Part model, mm, in its own coordinate system. Coordinates: 2 decimals unless noted, no trailing zeros. Loops run counter-clockwise (first coordinate to the right, second up) from the corner with the lowest first, then second, coordinate; pieces in that order, holes last. Notation, with made-up numbers: M -37.5,56.25 L 12.5,56.25 A18 cw 12.5,76.25 Z; hole C 32,75 d6. An arc over 180 degrees is marked long. Use a Markdown table: item, result. Add a question column.
1) Band-saw the part on A-A (y = 10). List the corners of the cut face in (x, z), plus the area to 3 significant figures.
2) Pin check, flat tips, straight feed: pin 1 Ø1.5 at (y, z) = (18.5, 2) entering from -X; pin 2 Ø1.5 at (y, z) = (9, 1.5) entering from +X; pin 3 Ø1.8 at (x, y) = (9.91, 15.79) entering from -Z. Stop position of each tip, or through.
3) Wall check: probe 1 along X at (y, z) = (25.25, 1.7); probe 2 along Y at (x, z) = (67.5, 0.1); probe 3 along Y at (x, z) = (19.5, 0.2). Give the ranges that are in metal, low to high. Write a range as from..to.
4) Band-saw the part on B-B (x = 15). List the corners of the cut face in (y, z), plus the area to 3 significant figures.
5) Band-saw the part on C-C (x = 33). List the corners of the cut face in (y, z), plus the area to 3 significant figures.
from build123d import *

# Parameters (mm, degrees)
MODEL_R                 = 1
SALIENTE_EXTRUIR1_DEPTH = 3


with BuildPart() as part:
    # Model → Saliente-Extruir1 (new body)
    with BuildSketch(Plane.XY):
        with BuildLine():
            Line((17.861622063, 18.20706488), (56.277425925, 14.846117598))
            Line((56.277425925, 14.846117598), (67.057874252, 21.223257456))
            ThreePointArc((67.057874252, 21.223257456), (71.209474737, 20.095027087), (69.964368376, 15.976969231))
            Line((69.964368376, 15.976969231), (55.736188762, 8.659748523))
            Line((55.736188762, 8.659748523), (18.934882774, 11.8794456))
            ThreePointArc((18.934882774, 11.8794456), (8.451096418, 6.06231898), (0.138961898, 14.702756365))
            Line((0.138961898, 14.702756365), (-1.772059081, 14.490982222))
            ThreePointArc((-1.772059081, 14.490982222), (-1.880981546, 14.481466547), (-1.990228383, 14.477019049))
            ThreePointArc((-1.990228383, 14.477019049), (-2.005285406, 14.476804272), (-2.020343495, 14.476685822))
            ThreePointArc((-2.020343495, 14.476685822), (-4.376324998, 17.035772608), (-1.611755391, 19.146869222))
            ThreePointArc((-1.611755391, 19.146869222), (-1.596946637, 19.144137761), (-1.582155659, 19.141311623))
            ThreePointArc((-1.582155659, 19.141311623), (-1.475340827, 19.117961178), (-1.369725519, 19.08967588))
            Line((-1.369725519, 19.08967588), (0.550429384, 18.527326068))
            ThreePointArc((0.550429384, 18.527326068), (1.632460158, 18.600931479), (2.408362946, 19.35868026))
            ThreePointArc((2.408362946, 19.35868026), (2.540100184, 19.623117729), (2.6811533, 19.882705658))
            ThreePointArc((2.6811533, 19.882705658), (2.856825208, 20.952914859), (2.296491875, 21.881480908))
            Line((2.296491875, 21.881480908), (0.734486272, 23.131829117))
            ThreePointArc((0.734486272, 23.131829117), (0.65073786, 23.202120333), (0.570343825, 23.276224656))
            ThreePointArc((0.570343825, 23.276224656), (0.559545032, 23.286719709), (0.548813598, 23.297283629))
            ThreePointArc((0.548813598, 23.297283629), (0.692430721, 26.772761747), (4.140047368, 26.310686561))
            ThreePointArc((4.140047368, 26.310686561), (4.148587304, 26.298283756), (4.157047724, 26.285826574))
            ThreePointArc((4.157047724, 26.285826574), (4.216065957, 26.193785825), (4.270746533, 26.099103798))
            Line((4.270746533, 26.099103798), (5.230859716, 24.343707882))
            ThreePointArc((5.230859716, 24.343707882), (6.048017899, 23.630643468), (7.132473325, 23.617806645))
            ThreePointArc((7.132473325, 23.617806645), (7.412611146, 23.711639877), (7.695907146, 23.795456646))
            ThreePointArc((7.695907146, 23.795456646), (8.576878126, 24.427990033), (8.837257977, 25.480800883))
            Line((8.837257977, 25.480800883), (8.602586519, 27.717719751))
            ThreePointArc((8.602586519, 27.717719751), (11.161673306, 30.073701254), (13.272769919, 27.309131647))
            Line((13.272769919, 27.309131647), (12.653226766, 25.146946875))
            ThreePointArc((12.653226766, 25.146946875), (12.726832176, 24.064916101), (13.484580957, 23.289013313))
            Line((13.484580957, 23.289013313), (14.008606355, 23.016222959))
            ThreePointArc((14.008606355, 23.016222959), (15.078815556, 22.840551052), (16.007381606, 23.400884385))
            Line((16.007381606, 23.400884385), (17.257729815, 24.962889987))
            ThreePointArc((17.257729815, 24.962889987), (17.328021031, 25.046638399), (17.402125353, 25.127032434))
            ThreePointArc((17.402125353, 25.127032434), (17.412620407, 25.137831227), (17.423184327, 25.148562661))
            ThreePointArc((17.423184327, 25.148562661), (20.898662444, 25.004945538), (20.436587259, 21.557328891))
            ThreePointArc((20.436587259, 21.557328891), (20.424184454, 21.548788955), (20.411727272, 21.540328535))
            ThreePointArc((20.411727272, 21.540328535), (20.319686522, 21.481310302), (20.225004495, 21.426629727))
            Line((20.225004495, 21.426629727), (18.46960858, 20.466516543))
            ThreePointArc((18.46960858, 20.466516543), (17.756544167, 19.64935836), (17.743707345, 18.564902935))
            ThreePointArc((17.743707345, 18.564902935), (17.804692888, 18.386652235), (17.861622063, 18.20706488))
        make_face()
        with Locations((9.911638477, 15.785737779)):
            Circle(MODEL_R, mode=Mode.SUBTRACT)
    extrude(amount=SALIENTE_EXTRUIR1_DEPTH)


solid = part.part
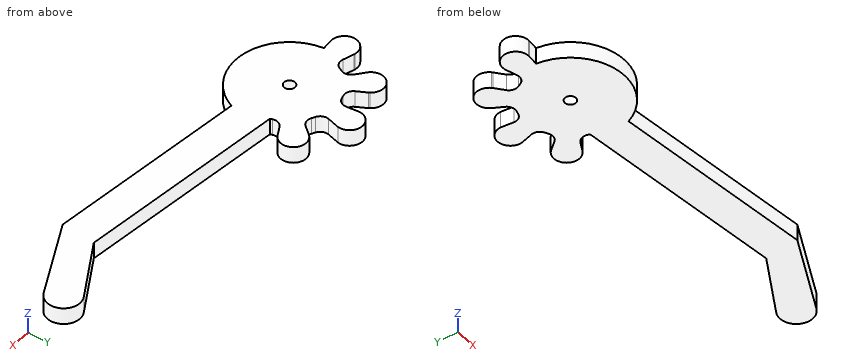
Entries:
| question | item | result |
|---|---|---|
| 1 | outline | M 1.96,0 L 17.86,0 L 17.86,3 L 1.96,3 Z; M 40.42,0 L 58.34,0 L 58.34,3 L 40.42,3 Z |
| 1 | area | 101 mm2 |
| 2 | pin 1 | x = -4.2 |
| 2 | pin 2 | x = 57.86 |
| 2 | pin 3 | through |
| 3 | probe 1 | -0.13..4.74, 8.85..12.68, 17.53..20.66 |
| 3 | probe 2 | 14.71..21.44 |
| 3 | probe 3 | 11.83..18.06, 21.03..25.81 |
| 4 | outline | M 7.37,0 L 22.83,0 L 22.83,3 L 7.37,3 Z |
| 4 | area | 46.4 mm2 |
| 5 | outline | M 10.65,0 L 16.88,0 L 16.88,3 L 10.65,3 Z |
| 5 | area | 18.7 mm2 |
